from build123d import *

# Parameters (mm, degrees)
BOSS_EXTRUDE1_DEPTH = 115
SKETCH2_W           = 40
SKETCH2_H           = 35
CUT_EXTRUDE1_DEPTH  = 41
CUT_EXTRUDE2_REACH  = 41.816
SKETCH4_W           = 15
SKETCH4_H           = 45
SKETCH4_H_2         = 40
BOSS_EXTRUDE2_DEPTH = 5
CUT_EXTRUDE3_DEPTH  = 15
SKETCH7_W           = 15
SKETCH7_H           = 15
BOSS_EXTRUDE3_DEPTH = 10
SKETCH8_W           = 15.002545061
SKETCH8_H           = 15
BOSS_EXTRUDE4_DEPTH = 10


with BuildPart() as part:
    # Sketch1 → Boss-Extrude1 (new body)
    with BuildSketch(Plane(origin=(0, 0, 0), x_dir=(1, 0, 0), z_dir=(0, 1, 0))):
        with BuildLine():
            Line((0, 0), (0, -15))
            Line((0, -15), (-40, -15))
            Line((-40, -15), (-40, -39.815551805))
            ThreePointArc((-40, -39.815551805), (-69.724211568, 11.254514819), (-30, 55))
            Line((-30, 55), (-30, 10))
            ThreePointArc((-30, 10), (-27.071067812, 2.928932188), (-20, 0))
            Line((-20, 0), (0, 0))
        make_face()
    extrude(amount=BOSS_EXTRUDE1_DEPTH)

    # Sketch2 → Cut-Extrude1 (cut, through all)
    with BuildSketch(Plane(origin=(-30, 0, 0), x_dir=(0, 0, -1), z_dir=(1, 0, 0))):
        with Locations((35, 52.5)):
            Rectangle(SKETCH2_W, SKETCH2_H)
    extrude(amount=-CUT_EXTRUDE1_DEPTH, mode=Mode.SUBTRACT)

    # Sketch3 → Cut-Extrude2 (cut, up to next)
    with BuildSketch(Plane(origin=(0, 0, 0), x_dir=(-1, 0, 0), z_dir=(0, 0, -1)), mode=Mode.PRIVATE) as cut_extrude2_sk1:
        with BuildLine():
            Line((15, 90), (15, 10))
            ThreePointArc((15, 10), (10, 5), (5, 10))
            Line((5, 10), (5, 90))
            ThreePointArc((5, 90), (10, 95), (15, 90))
        make_face()
    cut_extrude2_tool1 = extrude(cut_extrude2_sk1.sketch, amount=-CUT_EXTRUDE2_REACH, mode=Mode.PRIVATE) & part.part
    add(cut_extrude2_tool1.solids().sort_by_distance((-10, 50, 0))[0], mode=Mode.SUBTRACT)

    # Sketch4 → Boss-Extrude2 (add)
    with BuildSketch(Plane(origin=(-30, 0, 0), x_dir=(0, 0, -1), z_dir=(1, 0, 0))):
        with Locations((32.5, 12.5)):
            Rectangle(SKETCH4_W, SKETCH4_H)
        with Locations((32.5, 90)):
            Rectangle(SKETCH4_W, SKETCH4_H_2)
    extrude(amount=BOSS_EXTRUDE2_DEPTH)

    # Sketch6 → Cut-Extrude3 (cut)
    with BuildSketch(Plane(origin=(0, 115, 0), x_dir=(1, 0, 0), z_dir=(0, 1, 0))):
        with BuildLine():
            Line((0, -10), (-69.987139252, 4.87622568))
            ThreePointArc((-69.987139252, 4.87622568), (-59.085961763, 37.191731616), (-30, 55))
            Line((-30, 55), (-30, 10))
            ThreePointArc((-30, 10), (-27.071067812, 2.928932188), (-20, 0))
            Line((-20, 0), (0, 0))
            Line((0, 0), (0, -10))
        make_face()
    extrude(amount=-CUT_EXTRUDE3_DEPTH, mode=Mode.SUBTRACT)

    # Sketch7 → Boss-Extrude3 (add)
    with BuildSketch(Plane(origin=(0, 100, 0), x_dir=(1, 0, 0), z_dir=(0, 1, 0))):
        with Locations((-37.5, 32.5)):
            Rectangle(SKETCH7_W, SKETCH7_H)
    extrude(amount=BOSS_EXTRUDE3_DEPTH)

    # Sketch8 → Boss-Extrude4 (add)
    with BuildSketch(Plane.XZ):
        with Locations((-37.501272531, -32.5)):
            Rectangle(SKETCH8_W, SKETCH8_H)
    extrude(amount=BOSS_EXTRUDE4_DEPTH)


solid = part.part
Design review of the part built by this model. Coordinates are the model's own, in mm. A direction names the side the tool comes from. Round coordinates to 2 decimals unless told otherwise and drop trailing zeros. Write each loop counter-clockwise with the first axis right and the second up, starting at its lowest first coordinate (ties: lowest second). Pieces come first, ordered by that corner, then holes. Notation, with made-up numbers: M 23.25,8 L 54.25,8 A35 cw 54.25,47 Z; hole C 48.5,2 d9. An arc over 180 degrees is marked long. One line per item, written item: value. Start each with the question number.
1. Clearance check with flat-ended pins moving along their axes: P1, Ø5, axis at y = 91, z = -37.5, coming from the +X side; P2, Ø3, axis at x = -26.5, y = 42.5, coming from the +Z side; P3, Ø3, axis at y = 105.5, z = -33, coming from the -X side. State where each tip first meets the part, or that it passes through.
2. To check wall thickness, follow probe 1 along Y at (x, z) = (-52, -30); probe 2 along Z at (x, y) = (-18, 5); probe 3 along Z at (x, y) = (-27, 6.5). State the ranges of each line that lie inside material, in increasing order. Write a range as from..to.
3. Take a section at B-B on x = -10. State the section outline as (y, z) points, then the cut area to 3 significant figures.
4. Take a section at D-D on z = 1.5. State the section outline as (x, y) points, then the cut area to 3 significant figures.
5. Take a section at A-A on y = 72.5. State the section outline as (x, z) points.
6. Take a section at C-C on z = -27.5. State the section outline as (x, y) points.
7. Draft analysis for pull direction Y (two halves, no side actions). For faces 4 (the face through (-40, 57, 27)), 5 (the face through (-35, -10, -32)), 6 (the face through (-49, 52, -15)), 7 (the face through (-10, 5, 7)), state which applies: pulls with the +Y half, pulls with the -Y half, needs draft (parallel to the pull), parting line crosses it, or undercut.
8. For faces 1 (the face through (-28, 99, -25)), 2 (the face through (-42, 35, -30)), 3 (the face through (-5, 49, 7)), list the 3-axis set-ups (+Z, -Z, +X, -X, +Y, -Y) from which the entire face can be reached by the end or side of a thin tool; tool diameter is ignored.
Computed:
1. P1: stops at x = -25
1. P2: stops at z = 15
1. P3: stops at x = -45
2. probe 1: y = 0..35, 70..100
2. probe 2: z = 0..15
2. probe 3: z = -40..-25, -2.86..15
3. outline: M 0,0 L 5,0 L 5,15 L 0,15 Z; M 95,0 L 100,0 L 100,7.87 L 115,7.87 L 115,15 L 95,15 Z
3. area: 257 mm²
4. outline: M -69.43,0 L 0,0 L 0,100 L -39.99,100 L -39.99,115 L -69.43,115 Z; hole M -15,10 A5 ccw -5,10 L -5,90 A5 ccw -15,90 Z
4. area: 6,510 mm²
5. outline: M -40,15 L -40,39.82 A50 ccw -30,-55 L -30,-40 L -25,-40 L -25,-25 L -30,-25 L -30,-10 A10 cw -20,0 L -15,0 L -15,15 Z; M -5,0 L 0,0 L 0,15 L -5,15 Z
6. outline: M -65.15,0 L -45,0 L -45,-10 L -25,-10 L -25,35 L -65.15,35 Z; M -65.15,70 L -25,70 L -25,110 L -45,110 L -45,100 L -65.15,100 Z
7. face 4: needs draft
7. face 5: pulls with the -Y half
7. face 6: undercut
7. face 7: undercut
8. face 1: +X, +Y
8. face 2: -Z, +X, -X
8. face 3: +Z, -Z
